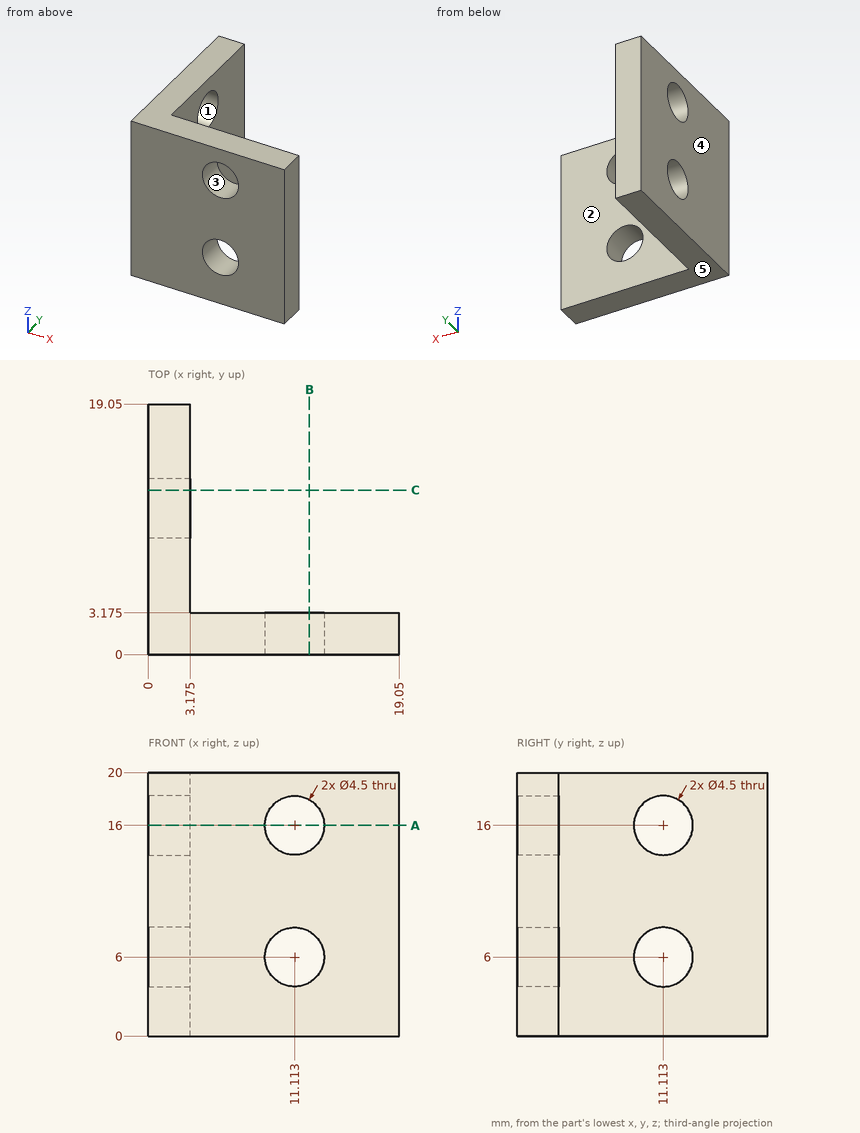
Verification items for this drawing (mm, ordinates from the low corner). A direction names the side the tool comes from. Coordinates: 2 decimals unless noted, no trailing zeros. Write each loop counter-clockwise with the first axis right and the second up, starting at its lowest first coordinate (ties: lowest second). Pieces come first, ordered by that corner, then holes. Notation, with made-up numbers: M 57,8.5 L 93,8.5 A8 ccw 93,18.5 Z; hole C 82.5,50.5 d11. An arc over 180 degrees is marked long. One line per item, written item: value. Start each with the question number.
(1) Sectioned sample at B-B, the plane x = 12.25. Enter the section's corners in (y, z) (1 decimal).
(2) Scan lines: line 1 along Y through (x, z) = (0.9, 6); line 2 along Y through (x, z) = (12.25, 19) (1 decimal). Record each from-to range of solid material in increasing order. Write a range as [from, to].
(3) Tool access check on the marked faces 1 and 2. Record the directions out of +Z, -Z, +X, -X, +Y, -Y that give a thin tool (end or side, any length) a straight path to the whole face; none if there is none.
(4) Sectioned sample at C-C, the plane y = 12.5. Enter the section's corners in (x, z) (1 decimal).
(5) Release check for a two-part mould opening along Z. For the marked faces 3, 4 and 5 record: released by +Z, released by -Z, zero draft, split by the parting line, or undercut.
(6) Sectioned sample at A-A, the plane z = 16. State how many separate pieces and enclosed holes the cut face has.
(7) Depth check by flat-ended pin: pin 1 (8 mm diameter, centred on x = 8, z = 15, fed in from +Y) (1 decimal); pin 2 (5 mm diameter, centred on x = 7, y = 10, fed in from +Z). Enter the tip coordinate at first touch or a pass-through.
Filled sheet:
1. outline: M 0,0 L 3.2,0 L 3.2,4.1 L 0,4.1 Z; M 0,7.9 L 3.2,7.9 L 3.2,14.1 L 0,14.1 Z; M 0,17.9 L 3.2,17.9 L 3.2,20 L 0,20 Z
2. line 1: [0, 8.86], [13.36, 19.05]
2. line 2: [0, 3.2]
3. face 1: +X, -X
3. face 2: +Z, -Z, +X, +Y
4. outline: M 0,0 L 3.2,0 L 3.2,4.2 L 0,4.2 Z; M 0,7.8 L 3.2,7.8 L 3.2,14.2 L 0,14.2 Z; M 0,17.8 L 3.2,17.8 L 3.2,20 L 0,20 Z
5. face 3: undercut
5. face 4: zero draft
5. face 5: released by -Z
6. separate pieces: 3
6. enclosed holes: 0
7. pin 1: y = 3.2
7. pin 2: through
